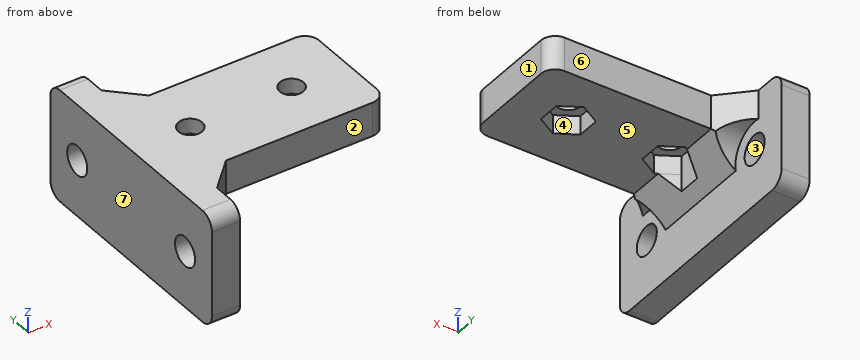
```python
from build123d import *

# Parameters (mm, degrees)
SKETCH_1_W          = 38.5
SKETCH_1_H          = 20
EXTRUDE_1_DEPTH     = 6
SKETCH_2_W          = 20
SKETCH_2_H          = 42
EXTRUDE_2_DEPTH     = 5
SKETCH_3_R          = 2.1
CUT_EXTRUDE_1_DEPTH = 35.807506374
CUT_EXTRUDE_2_DEPTH = 3.3
SKETCH_5_R          = 2.6
CUT_EXTRUDE_3_DEPTH = 42.943414263
CHAMFER_2_SIZE      = 5
SKETCH_6_R          = 5
CUT_EXTRUDE_4_DEPTH = 42.943414263
FILLET_1_R          = 2.5


with BuildPart() as part:
    # Эскиз1 → Бобышка-Вытянуть1 (new body)
    with BuildSketch(Plane.XY):
        Rectangle(SKETCH_1_W, SKETCH_1_H)
    extrude(amount=EXTRUDE_1_DEPTH)

    # Эскиз2 → Бобышка-Вытянуть2 (add)
    with BuildSketch(Plane.ZY.offset(19.25)):
        with Locations((-4, 0)):
            Rectangle(SKETCH_2_W, SKETCH_2_H)
    extrude(amount=-EXTRUDE_2_DEPTH)

    # Эскиз3 → Вырез-Вытянуть1 (cut, through all)
    with BuildSketch(Plane.XY.offset(6)):
        with Locations((9.25, 0)):
            Circle(SKETCH_3_R)
        with Locations((-8.75, 0)):
            Circle(SKETCH_3_R)
    extrude(amount=-CUT_EXTRUDE_1_DEPTH, mode=Mode.SUBTRACT)

    # Эскиз4 → Вырез-Вытянуть2 (cut)
    with BuildSketch(Plane(origin=(0, 0, 0), x_dir=(-1, 0, 0), z_dir=(0, 0, -1))):
        Polygon((8.75, 4.041451884), (5.25, 2.020725942), (5.25, -2.020725942), (8.75, -4.041451884), (12.25, -2.020725942), (12.25, 2.020725942), align=None)
        Polygon((-9.25, 4.041451884), (-12.75, 2.020725942), (-12.75, -2.020725942), (-9.25, -4.041451884), (-5.75, -2.020725942), (-5.75, 2.020725942), align=None)
    extrude(amount=-CUT_EXTRUDE_2_DEPTH, mode=Mode.SUBTRACT)

    # Эскиз5 → Вырез-Вытянуть3 (cut, through all)
    with BuildSketch(Plane(origin=(-14.25, 0, 0), x_dir=(0, 0, -1), z_dir=(1, 0, 0))):
        with Locations((4, 14)):
            Circle(SKETCH_5_R)
        with Locations((4, -14)):
            Circle(SKETCH_5_R)
    extrude(amount=-CUT_EXTRUDE_3_DEPTH, mode=Mode.SUBTRACT)

    # Фаска2
    # the kernel refuses this chamfer: 5 mm, written as the material it adds along each edge
    with BuildSketch(Plane(origin=(-14.25, 10, -12.85841494), x_dir=(0, 1, 0), z_dir=(0, 0, 1))) as chamfer_2_piece_1_section:
        Polygon((CHAMFER_2_SIZE, 0), (0, -CHAMFER_2_SIZE), (0, 0), align=None)
    chamfer_2_piece_1 = extrude(amount=18.85841494, mode=Mode.PRIVATE)
    chamfer_2_piece_1 = chamfer_2_piece_1 - Plane(origin=(-14.25, 14, -4), x_dir=(0, 0, -1), z_dir=(1, 0, 0)) * Cylinder(2.6, 58, mode=Mode.PRIVATE)
    chamfer_2_piece_1 = split(chamfer_2_piece_1, bisect_by=Plane(origin=(-18.17920747, 10, -8.92920747), z_dir=(-0.7071067811865476, 0, 0.7071067811865476)), keep=Keep.TOP, mode=Mode.PRIVATE)
    add(chamfer_2_piece_1)
    with BuildSketch(Plane(origin=(-14.25, -10, 6), x_dir=(0, -1, 0), z_dir=(0, 0, -1))) as chamfer_2_piece_2_section:
        Polygon((CHAMFER_2_SIZE, 0), (0, -CHAMFER_2_SIZE), (0, 0), align=None)
    chamfer_2_piece_2 = extrude(amount=18.85841494, mode=Mode.PRIVATE)
    chamfer_2_piece_2 = chamfer_2_piece_2 - Plane(origin=(-14.25, -14, -4), x_dir=(0, 0, -1), z_dir=(1, 0, 0)) * Cylinder(2.6, 58, mode=Mode.PRIVATE)
    chamfer_2_piece_2 = split(chamfer_2_piece_2, bisect_by=Plane(origin=(-8.75, -10, 0.5), z_dir=(-0.7071067811865476, 0, 0.7071067811865476)), keep=Keep.TOP, mode=Mode.PRIVATE)
    add(chamfer_2_piece_2)
    with BuildSketch(Plane(origin=(-14.25, -22.85841494, 0), x_dir=(0, 0, -1), z_dir=(0, 1, 0))) as chamfer_2_piece_3_section:
        Polygon((CHAMFER_2_SIZE, 0), (0, -CHAMFER_2_SIZE), (0, 0), align=None)
    chamfer_2_piece_3 = extrude(amount=45.71682988, mode=Mode.PRIVATE)
    chamfer_2_piece_3 = chamfer_2_piece_3 - Plane(origin=(-14.25, -14, -4), x_dir=(0, 0, -1), z_dir=(1, 0, 0)) * Cylinder(2.6, 112, mode=Mode.PRIVATE)
    chamfer_2_piece_3 = split(chamfer_2_piece_3, bisect_by=Plane(origin=(-4.727015986, -6.364122788, 0), z_dir=(-0.5, -0.8660254037844387, 0)), keep=Keep.TOP, mode=Mode.PRIVATE)
    chamfer_2_piece_3 = split(chamfer_2_piece_3, bisect_by=Plane(origin=(-18.17920747, -18.92920747, 0), z_dir=(-0.7071067811865478, 0.7071067811865472, 0)), keep=Keep.TOP, mode=Mode.PRIVATE)
    add(chamfer_2_piece_3)
    with BuildSketch(Plane(origin=(-14.25, -22.85841494, 0), x_dir=(0, 0, -1), z_dir=(0, 1, 0))) as chamfer_2_piece_4_section:
        Polygon((CHAMFER_2_SIZE, 0), (0, -CHAMFER_2_SIZE), (0, 0), align=None)
    chamfer_2_piece_4 = extrude(amount=45.71682988, mode=Mode.PRIVATE)
    chamfer_2_piece_4 = chamfer_2_piece_4 - Plane(origin=(-14.25, 14, -4), x_dir=(0, 0, -1), z_dir=(1, 0, 0)) * Cylinder(2.6, 112, mode=Mode.PRIVATE)
    chamfer_2_piece_4 = split(chamfer_2_piece_4, bisect_by=Plane(origin=(-4.727015986, -6.364122788, 0), z_dir=(0.5, 0.8660254037844387, 0)), keep=Keep.TOP, mode=Mode.PRIVATE)
    chamfer_2_piece_4 = split(chamfer_2_piece_4, bisect_by=Plane(origin=(-12.25, -22.85841494, 0), z_dir=(-1, 0, 0)), keep=Keep.TOP, mode=Mode.PRIVATE)
    chamfer_2_piece_4 = split(chamfer_2_piece_4, bisect_by=Plane(origin=(4.67920747, -3.92920747, 0), z_dir=(-0.7071067811865476, -0.7071067811865476, 0)), keep=Keep.TOP, mode=Mode.PRIVATE)
    add(chamfer_2_piece_4)
    with BuildSketch(Plane(origin=(-14.25, -22.85841494, 0), x_dir=(0, 0, -1), z_dir=(0, 1, 0))) as chamfer_2_piece_5_section:
        Polygon((CHAMFER_2_SIZE, 0), (0, -CHAMFER_2_SIZE), (0, 0), align=None)
    chamfer_2_piece_5 = extrude(amount=45.71682988, mode=Mode.PRIVATE)
    chamfer_2_piece_5 = chamfer_2_piece_5 - Plane(origin=(-14.25, 14, -4), x_dir=(0, 0, -1), z_dir=(1, 0, 0)) * Cylinder(2.6, 112, mode=Mode.PRIVATE)
    chamfer_2_piece_5 = split(chamfer_2_piece_5, bisect_by=Plane(origin=(-24.522984014, -5.065084682, 0), z_dir=(-0.4999999999999998, 0.8660254037844388, 0)), keep=Keep.TOP, mode=Mode.PRIVATE)
    chamfer_2_piece_5 = split(chamfer_2_piece_5, bisect_by=Plane(origin=(4.67920747, -3.92920747, 0), z_dir=(-0.7071067811865476, -0.7071067811865476, 0)), keep=Keep.TOP, mode=Mode.PRIVATE)
    add(chamfer_2_piece_5)

    # Эскиз6 → Вырез-Вытянуть4 (cut, through all)
    with BuildSketch(Plane(origin=(-14.25, 0, 0), x_dir=(0, 0, -1), z_dir=(1, 0, 0))):
        with Locations((4, -14)):
            Circle(SKETCH_6_R)
        with Locations((4, 14)):
            Circle(SKETCH_6_R)
    extrude(amount=CUT_EXTRUDE_4_DEPTH, mode=Mode.SUBTRACT)

    # Скругление1
    fillet_1_edges = [part.edges().sort_by_distance(p)[0] for p in [
        (-16.75, 21, 6),
        (-16.75, -21, 6),
        (-16.75, -21, -14),
        (-16.75, 21, -14),
        (19.25, 10, 3),
        (19.25, -10, 3),
    ]]
    fillet(fillet_1_edges, radius=FILLET_1_R)


solid = part.part
```
Verification items for the finished model (mm, model axes). Face numbers are marked on the shaded views. A direction names the side the tool comes from. Coordinates: 2 decimals unless noted, no trailing zeros. Write each loop counter-clockwise with the first axis right and the second up, starting at its lowest first coordinate (ties: lowest second). Pieces come first, ordered by that corner, then holes. Notation, with made-up numbers: (81, -4.5) - (123, -4.5) arc R20 ccw to (123, -0.5) - close; hole circle Ø11 at (26, 79). An arc over 180 degrees is marked (long way). Write item = value, one per line.
Q1. Go/stop test with flat-tipped pins: pin 1 Ø2 at (x, y) = (8.5, -2) entering from -Z; pin 2 Ø8.5 at (y, z) = (14, -4) entering from +X; pin 3 Ø6.5 at (x, z) = (0, 2) entering from +Y. Record where each tip stops, or that it passes through.
Answer:
pin_1 = 3.3
pin_2 = -14.25
pin_3 = 10
Q2. Mould release check, pull along Y, two halves, no side actions. Record for the marked faces 1, 2 and 3: released by +Y, released by -Y, zero draft, split by the parting line, or undercut.
Answer:
face_1 = zero draft
face_2 = released by -Y
face_3 = undercut
Q3. Cross-section at D-D (z = -4). Enter the section's corners in (x, y).
Answer:
outline = (-19.25, -21) - (-14.25, -21) - (-14.25, -16.6) - (-19.25, -16.6) - close; (-19.25, -11.4) - (-14.25, -11.4) - (-14.25, -9) - (-13.25, -9) - (-13.25, 9) - (-14.25, 9) - (-14.25, 11.4) - (-19.25, 11.4) - close; (-19.25, 16.6) - (-14.25, 16.6) - (-14.25, 21) - (-19.25, 21) - close
Q4. Access from +Z, -Z, +X, -X, +Y, -Y to the whole of each face (thin tool, end or side, straight path). Record for the marked faces 4, 5, 6 and 7.
Answer:
face_4 = -Z
face_5 = -Z, +X, +Y, -Y
face_6 = +Z, -Z, +X, +Y
face_7 = +Z, -Z, -X, +Y, -Y
Q5. Material ranges on L1, parallel to Y at x = -15.95, z = -4; L2, parallel to Z at x = -17.3, y = -14; L3, parallel to Y at x = -8.75, z = 5.2, recorded low to high. Write a range as from..to.
Answer:
L1 = -21..-16.6, -11.4..11.4, 16.6..21
L2 = -14..-6.6, -1.4..6
L3 = -10..-2.1, 2.1..10
Q6. Cross-section at C-C (x = -8). Enter the section's corners in (y, z), plus the area to 3 significant figures.
Answer:
outline = (-10, 0) - (-3.61, 0) - (-3.61, 3.3) - (-1.96, 3.3) - (-1.96, 6) - (-10, 6) - close; (1.96, 3.3) - (3.61, 3.3) - (3.61, 0) - (10, 0) - (10, 6) - (1.96, 6) - close
area = 85.6 mm²
Q7. Cross-section at B-B (z = 2.75). Enter the section's corners in (x, y).
Answer:
outline = (-19.25, -21) - (-14.25, -21) - (-14.25, -15) - (-9.25, -10) - (16.75, -10) arc R2.5 ccw to (19.25, -7.5) - (19.25, 7.5) arc R2.5 ccw to (16.75, 10) - (-9.25, 10) - (-14.25, 15) - (-14.25, 21) - (-19.25, 21) - close; hole (-12.25, -2.02) - (-8.75, -4.04) - (-5.25, -2.02) - (-5.25, 2.02) - (-8.75, 4.04) - (-12.25, 2.02) - close; hole (5.75, -2.02) - (9.25, -4.04) - (12.75, -2.02) - (12.75, 2.02) - (9.25, 4.04) - (5.75, 2.02) - close
Q8. Cross-section at A-A (y = 0). Enter the section's corners in (x, z), plus the area to 3 significant figures.
Answer:
outline = (-19.25, -14) - (-14.25, -14) - (-14.25, -5) - (-12.25, -3) - (-12.25, 3.3) - (-10.85, 3.3) - (-10.85, 6) - (-19.25, 6) - close; (-6.65, 3.3) - (-5.25, 3.3) - (-5.25, 0) - (5.75, 0) - (5.75, 3.3) - (7.15, 3.3) - (7.15, 6) - (-6.65, 6) - close; (11.35, 3.3) - (12.75, 3.3) - (12.75, 0) - (19.25, 0) - (19.25, 6) - (11.35, 6) - close
area = 240 mm²
